```python
from build123d import *

# Parameters (mm, degrees)
F0_W     = 67.357816
F0_H     = 43.378917
F1_DEPTH = 50.8
F2_R     = 9.927663
F3_DEPTH = 50.8
F2_R_2   = 13.600689
F4_DEPTH = 12.7


with BuildPart() as f1:
    # F0 (on Front) → F1 (new body)
    with BuildSketch(Plane.XZ):
        with Locations((-33.678908, 23.978901)):
            Rectangle(F0_W, F0_H)
    extrude(amount=F1_DEPTH)

    # F2 (on face) → F3 (cut)
    with BuildSketch(Plane(origin=(0, 0, 0), x_dir=(-1, 0, 0), z_dir=(0, 1, 0))):
        with Locations((34.82363, 23.737906)):
            Circle(F2_R)
    extrude(amount=-F3_DEPTH, mode=Mode.SUBTRACT)

    # F2 (on face) → F4 (join)
    with BuildSketch(Plane(origin=(0, 0, 0), x_dir=(-1, 0, 0), z_dir=(0, 1, 0))):
        with Locations((34.82363, 23.737906)):
            Circle(F2_R_2)
        with Locations((34.82363, 23.737906)):
            Circle(F2_R, mode=Mode.SUBTRACT)
    extrude(amount=F4_DEPTH)


solid = f1.part
```
The listing builds one solid part. Answer for the finished solid, in the listing's coordinates (mm). A direction names the side the tool comes from. Give positions to 0.01 mm unless a question says otherwise; leave off trailing zeros. Write each loop counter-clockwise with the first axis right and the second up, starting at its lowest first coordinate (ties: lowest second). Pieces come first, ordered by that corner, then holes. Notation, with made-up numbers: (62.5, 15.25) - (86.5, 15.25) arc R21 cw to (86.5, 54.25) - close; hole circle Ø6 at (-19.75, -37). An arc over 180 degrees is marked (long way). Use one line per item in the form item = value. Start each with the question number.
1) Flat-ended cylindrical pins translate along their axes: pin 1 Ø10 at (x, z) = (-11, 8.5) entering from +Y; pin 2 Ø18 at (x, z) = (-34.82, 23.74) entering from -Y; pin 3 Ø1.5 at (y, z) = (-18, 38.5) entering from +X. Find the tip coordinate at first contact, or state that the pin passes through.
2) Find section A-A on z = 20. Determine the outline of the cut face in (x, y), plus the area to 3 significant figures.
3) Consider line 1 along Y through (x, z) = (-46, 12); line 2 along X through (y, z) = (-43, 18); line 3 along X through (y, z) = (-42.5, 28.5). Determine where each line is inside the solid, lowest interval first. Write a range as from..to.
4) The mould has two halves that part along Z. Classify faces 1 (the face through (-27.51, -19.49, 30.45)), 2 (the face through (-34, -25, 2.289)), 3 (the face through (-34, -25, 45.668)), 4 (the face through (-34, -50.8, 34)): pulls with the +Z half, pulls with the -Z half, needs draft (parallel to the pull), parting line crosses it, or undercut.
5) Find section C-C on x = -46. Determine the outline of the cut face in (y, z), plus the area to 3 significant figures.
6) Find section B-B on x = -31. Determine the outline of the cut face in (y, z), plus the area to 3 significant figures.
7) Find section D-D on y = -2.5. Determine the outline of the cut face in (x, z), plus the area to 3 significant figures.
8) A tool of negligible diameter and unlimited length cuts with its end or side. For faces 5 (the face through (-21.236, 6.261, 24.336)), 6 (the face through (-67.358, -25, 24)), from which of +Z, -Z, +X, -X, +Y, -Y can it reach the whole face along a straight path? Write none if from no direction.
Geometry results:
q1.pin_1 = 0
q1.pin_2 = through
q1.pin_3 = 0
q2.outline = (-67.36, -50.8) - (-44.02, -50.8) - (-44.02, 12.7) - (-47.9, 12.7) - (-47.9, 0) - (-67.36, 0) - close; (-25.63, -50.8) - (0, -50.8) - (0, 0) - (-21.75, 0) - (-21.75, 12.7) - (-25.63, 12.7) - close
q2.area = 2,590 mm2
q3.line_1 = -50.8..0
q3.line_2 = -67.36..-42.93, -26.72..0
q3.line_3 = -67.36..-43.53, -26.11..0
q4.face_1 = undercut
q4.face_2 = pulls with the -Z half
q4.face_3 = pulls with the +Z half
q4.face_4 = needs draft
q5.outline = (-50.8, 2.29) - (0, 2.29) - (0, 15.99) - (12.7, 15.99) - (12.7, 31.49) - (0, 31.49) - (0, 45.67) - (-50.8, 45.67) - close
q5.area = 2,400 mm2
q6.outline = (-50.8, 2.29) - (0, 2.29) - (0, 10.69) - (12.7, 10.69) - (12.7, 14.58) - (-50.8, 14.58) - close; (-50.8, 32.9) - (12.7, 32.9) - (12.7, 36.79) - (0, 36.79) - (0, 45.67) - (-50.8, 45.67) - close
q6.area = 1,370 mm2
q7.outline = (-67.36, 2.29) - (0, 2.29) - (0, 45.67) - (-67.36, 45.67) - close; hole circle Ø19.86 at (-34.82, 23.74)
q7.area = 2,610 mm2
q8.face_5 = +Y
q8.face_6 = +Z, -Z, -X, +Y, -Y
